```python
from build123d import *

# Parameters (mm, degrees)
F0_W     = 50.8
F0_H     = 38.1
F1_DEPTH = 31.75
F3_DEPTH = 50.801
F4_W     = 25.4
F4_H     = 19.05
F5_DEPTH = 25.4


with BuildPart() as f1:
    # F0 (on Front) → F1 (new body)
    with BuildSketch(Plane.XZ):
        with Locations((-25.4, 19.05)):
            Rectangle(F0_W, F0_H)
    extrude(amount=F1_DEPTH)

    # F2 (on face) → F3 (cut, through all)
    with BuildSketch(Plane.YZ):
        with BuildLine():
            Line((-31.75, 38.1), (-31.75, 12.7))
            ThreePointArc((-31.75, 12.7), (-13.916344, 20.266344), (-6.35, 38.1))
            Line((-6.35, 38.1), (-31.75, 38.1))
        make_face()
    extrude(amount=-F3_DEPTH, mode=Mode.SUBTRACT)

    # F4 (on face) → F5 (cut)
    with BuildSketch(Plane(origin=(0, 0, 0), x_dir=(-1, 0, 0), z_dir=(0, 1, 0))):
        with Locations((25.4, 28.575)):
            Rectangle(F4_W, F4_H)
    extrude(amount=-F5_DEPTH, mode=Mode.SUBTRACT)


solid = f1.part
```
Geometry check sheet. Reference: the model listing, model coordinates, mm. A direction names the side the tool comes from. Round coordinates to 2 decimals unless told otherwise and drop trailing zeros. Loops run counter-clockwise (first coordinate to the right, second up) from the corner with the lowest first, then second, coordinate; pieces in that order, holes last. Notation, with made-up numbers: (-37.5, 85.5) -> (-19.5, 85.5) arc R20 cw to (-19.5, 122.5) -> close; hole circle Ø5 at (33, 53.5). An arc over 180 degrees is marked (long way). Use a Markdown table: item, result.
(1) Go/stop test with flat-tipped pins: P1, Ø8, axis at x = -9.5, z = 23.5, coming from the -Y side; P2, Ø12, axis at x = -22, y = -4.5, coming from the +Z side. Record where each tip stops, or that it passes through.
Calculated:
| item | result |
|---|---|
| P1 | y = -14.72 |
| P2 | z = 19.05 |
(2) Sectioned sample at D-D (z = 31.5). Enter the section's corners in (x, y).
Calculated:
| item | result |
|---|---|
| outline | (-50.8, -7.32) -> (-38.1, -7.32) -> (-38.1, 0) -> (-50.8, 0) -> close; (-12.7, -7.32) -> (0, -7.32) -> (0, 0) -> (-12.7, 0) -> close |
(3) Set-up check for faces 1 (the flat face through (-25, -8, 19.05)), 2 (the flat face through (-50.8, -12, 15)): record each of +Z, -Z, +X, -X, +Y, -Y from which the full face is reachable in a straight line by a thin tool's end or side.
Calculated:
| item | result |
|---|---|
| face 1 | +Z, +Y, -Y |
| face 2 | +Z, -Z, -X, +Y, -Y |
(4) Sectioned sample at C-C (x = -39). Enter the section's corners in (y, z), then the cut area to 3 significant figures.
Calculated:
| item | result |
|---|---|
| outline | (-31.75, 0) -> (0, 0) -> (0, 38.1) -> (-6.35, 38.1) arc R25.85 cw to (-31.75, 12.7) -> close |
| area | 708 mm² |
(5) Scan lines: probe 1 along X at (y, z) = (-6, 34.5); probe 2 along Z at (x, y) = (-25, -12.5); probe 3 along Y at (x, z) = (-3.5, 31.5). Record each from-to range of solid material in increasing order.
Calculated:
| item | result |
|---|---|
| probe 1 | -50.8 to -38.1, -12.7 to 0 |
| probe 2 | 0 to 19.05 |
| probe 3 | -7.32 to 0 |
(6) Sectioned sample at A-A (z = 24). Enter the section's corners in (x, y), then the cut area to 3 significant figures.
Calculated:
| item | result |
|---|---|
| outline | (-50.8, -10.83) -> (-38.1, -10.83) -> (-38.1, 0) -> (-50.8, 0) -> close; (-12.7, -10.83) -> (0, -10.83) -> (0, 0) -> (-12.7, 0) -> close |
| area | 275 mm² |
(7) Sectioned sample at B-B (y = -3.5). Enter the section's corners in (x, z), then the cut area to 3 significant figures.
Calculated:
| item | result |
|---|---|
| outline | (-50.8, 0) -> (0, 0) -> (0, 38.1) -> (-12.7, 38.1) -> (-12.7, 19.05) -> (-38.1, 19.05) -> (-38.1, 38.1) -> (-50.8, 38.1) -> close |
| area | 1,450 mm² |
